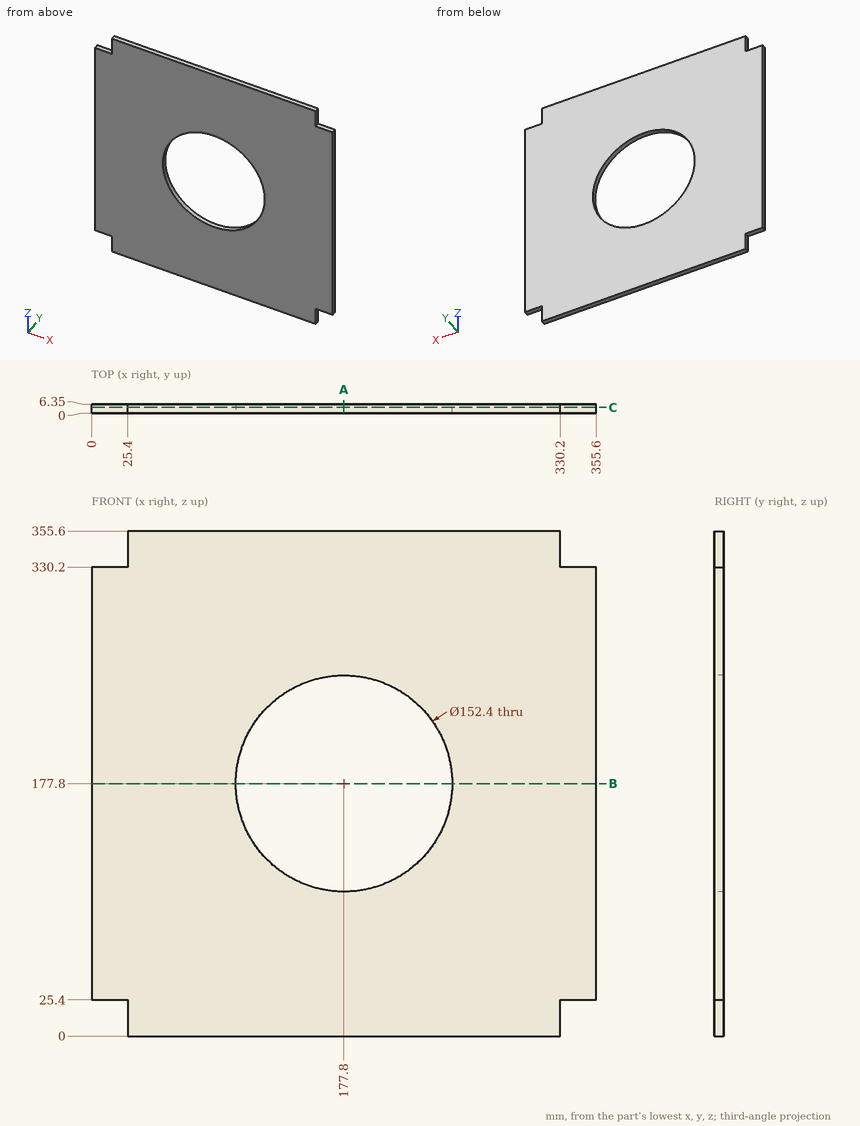
Input: dimensioned drawing with shaded views. Units: mm. Origin: part minimum x, y, z. Round coordinates to 2 decimals unless told otherwise and drop trailing zeros. Loops run counter-clockwise (first coordinate to the right, second up) from the corner with the lowest first, then second, coordinate; pieces in that order, holes last. Notation, with made-up numbers: (-35, -10) -> (-8, -10) arc R30 cw to (-8, 27) -> close; hole circle Ø9 at (70.5, 61.25). An arc over 180 degrees is marked (long way). Answer as a JSON object with one key per item and string values. Group by question number.
1) Pin query (flat end, axial travel): pin 1 (1.9 mm diameter, centred on y = 3, z = 346, fed in from +X); pin 2 (1.9 mm diameter, centred on y = 3, z = 338, fed in from -X); pin 3 (3 mm diameter, centred on x = 127, z = 277, fed in from -Y); pin 4 (3 mm diameter, centred on x = 338.5, y = 2.5, fed in from +Z). Return the tip coordinate at first contact, or that it passes through.
2) Section query C-C on y = 4. Output: boundary loops of the cut face in (x, z).
3) Section query B-B on z = 177.8. Output: boundary loops of the cut face in (x, y).
4) Ray query, L1, parallel to X at y = 4.25, z = 177.8; L2, parallel to Z at x = 17.5, y = 5.25. Return the intervals inside material, ascending.
5) Section query A-A on x = 177.8. Output: boundary loops of the cut face in (y, z).
Reply:
{
 "1": {"pin 1": "stops at x = 330.2", "pin 2": "stops at x = 25.4", "pin 3": "stops at y = 0", "pin 4": "stops at z = 330.2"},
 "2": {"outline": "(0, 25.4) -> (25.4, 25.4) -> (25.4, 0) -> (330.2, 0) -> (330.2, 25.4) -> (355.6, 25.4) -> (355.6, 330.2) -> (330.2, 330.2) -> (330.2, 355.6) -> (25.4, 355.6) -> (25.4, 330.2) -> (0, 330.2) -> close; hole circle Ø152.4 at (177.8, 177.8)"},
 "3": {"outline": "(0, 0) -> (101.6, 0) -> (101.6, 6.35) -> (0, 6.35) -> close; (254, 0) -> (355.6, 0) -> (355.6, 6.35) -> (254, 6.35) -> close"},
 "4": {"L1": "x = 0 to 101.6, 254 to 355.6", "L2": "z = 25.4 to 330.2"},
 "5": {"outline": "(0, 0) -> (6.35, 0) -> (6.35, 101.6) -> (0, 101.6) -> close; (0, 254) -> (6.35, 254) -> (6.35, 355.6) -> (0, 355.6) -> close"}
}
